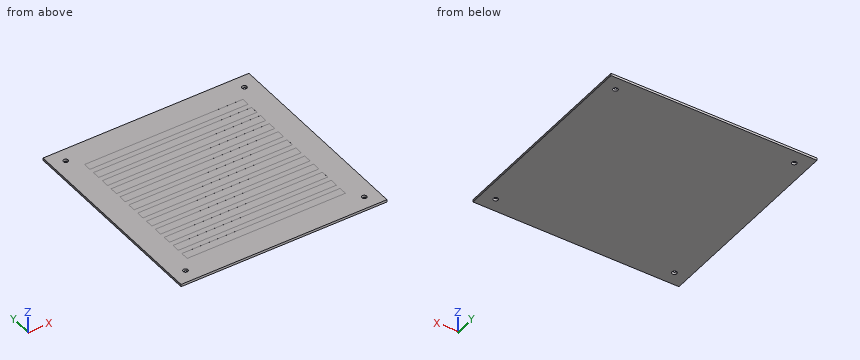
from build123d import *

# Parameters (mm, degrees)
SKETCH007_W            = 259.2
SKETCH007_H            = 259.2
PAD004_DEPTH           = 3
SKETCH008_W            = 199.2
SKETCH008_H            = 10
POCKET003_DEPTH        = 9.01
LINEARPATTERN005_COUNT = 12
LINEARPATTERN005_PITCH = 16.6
SKETCH013_R            = 3
POCKET008_DEPTH        = 12.001


with BuildPart() as part:
    # Sketch007 → Pad004 (new body)
    with BuildSketch(Plane.XY.offset(-9)):
        Rectangle(SKETCH007_W, SKETCH007_H)
    extrude(amount=-PAD004_DEPTH)

    # Sketch008 → Pocket003 (cut)
    with BuildSketch(Plane.XY):
        with Locations((0, 91.3)):
            Rectangle(SKETCH008_W, SKETCH008_H)
    pocket003 = extrude(amount=-POCKET003_DEPTH, mode=Mode.SUBTRACT)

    # LinearPattern005: Pocket003 ×12
    with Locations(*[(0, -i * LINEARPATTERN005_PITCH, 0) for i in range(1, LINEARPATTERN005_COUNT)]):
        add(pocket003, mode=Mode.SUBTRACT)

    # Sketch013 → Pocket008 (cut, through all)
    with BuildSketch(Plane.XY):
        with Locations((-112.5, 112.5)):
            Circle(SKETCH013_R)
        with Locations((112.5, 112.5)):
            Circle(SKETCH013_R)
        with Locations((112.5, -112.5)):
            Circle(SKETCH013_R)
        with Locations((-112.5, -112.5)):
            Circle(SKETCH013_R)
    extrude(amount=-POCKET008_DEPTH, mode=Mode.SUBTRACT)


solid = part.part
Model file for the job. Use its own axes, mm. Give positions to 0.01 mm unless a question says otherwise; leave off trailing zeros. Loops run counter-clockwise (first coordinate to the right, second up) from the corner with the lowest first, then second, coordinate; pieces in that order, holes last.
Item 1: Drop a flat-ended pin along its axis: P1, Ø3, axis at x = 36, y = -59, coming from the +Z side. Give the stop position or say it passes through.
Check values:
P1: stops at z = -9.01
Item 2: Drill centre lines: line 1 along Y through (x, z) = (-112.5, -11.2); line 2 along Z through (x, y) = (42.5, -90). Where is each one in solid material? Low to high.
Check values:
line 1: y = -129.6 to -115.5, -109.5 to 109.5, 115.5 to 129.6
line 2: z = -12 to -9.01
Item 3: Slice it at A-A (x = 112.5). Write the cut outline in (y, z).
Check values:
outline: (-129.6, -12) - (-115.5, -12) - (-115.5, -9) - (-129.6, -9) - close; (-109.5, -12) - (109.5, -12) - (109.5, -9) - (-109.5, -9) - close; (115.5, -12) - (129.6, -12) - (129.6, -9) - (115.5, -9) - close
